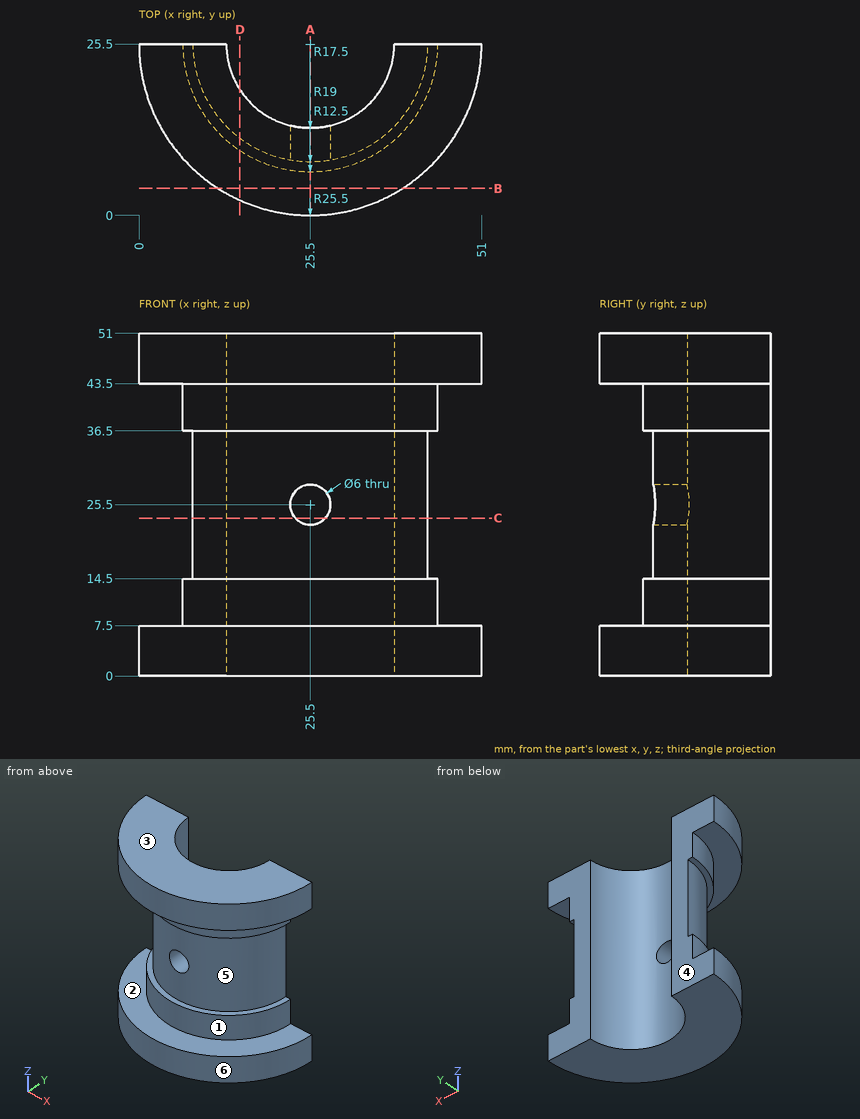
Here's the drawing with two shaded views (mm, measured from the low corner). I have some questions. A direction names the side the tool comes from. Coordinates: 2 decimals unless noted, no trailing zeros. Write each loop counter-clockwise with the first axis right and the second up, starting at its lowest first coordinate (ties: lowest second). Pieces come first, ordered by that corner, then holes.
Item 1: On a 3-axis mill with a long thin cutter (end or side, diameter ignored), from which of +Z, -Z, +X, -X, +Y, -Y can I reach the whole of each face in a straight line? I mean the marked faces 5 and 6. Say none if no direction works.
Item 2: If I drill on line 1 (Z direction, x = 7, y = 8.5); line 2 (Z direction, x = 25.5, y = 11.85); line 3 (Y direction, x = 2.5, z = 5), over which ranges is the centre line in solid material (lowest first)?
Item 3: If we mould it in two halves opening along Z, with no side actions, what happens to the marked faces 1, 2, 3 and 4? For each: +Z half, -Z half, draft (parallel to the pull), parting line (faces both ways), or undercut.
Item 4: I want a section at B-B on y = 4. Write out the boundary of the cut face in (x, z).
Item 5: I want a section at D-D on x = 15. Write out the boundary of the cut face in (y, z), and give its area (3 significant figures).
Item 6: Will these pins go through, and if not, where does the flat tip stop? pin 1 (2 mm diameter, centred on x = 19, z = 31.5, fed in from -Y); pin 2 (8 mm diameter, centred on y = 21, z = 41, fed in from +X); pin 3 (6 mm diameter, centred on x = 45.5, z = 36, fed in from -Y).
Item 7: I want a section at C-C on z = 23.5. Write out the boundary of the cut face in (x, y), and give its area (3 significant figures).
Item 8: I want a section at A-A on x = 25.5. Write out the boundary of the cut face in (y, z).
Findings below:
1. face 5: -Y
1. face 6: +Z, -Z, -Y
2. line 1: z = 0 to 7.5, 43.5 to 51
2. line 2: z = 0 to 22.5, 28.5 to 51
2. line 3: y = 14.49 to 25.5
3. face 1: undercut
3. face 2: undercut
3. face 3: +Z half
3. face 4: draft
4. outline: (11.79, 0) - (39.21, 0) - (39.21, 7.5) - (11.79, 7.5) - close; (11.79, 43.5) - (39.21, 43.5) - (39.21, 51) - (11.79, 51) - close
5. outline: (2.26, 0) - (18.72, 0) - (18.72, 51) - (2.26, 51) - (2.26, 43.5) - (9.66, 43.5) - (9.66, 36.5) - (11.5, 36.5) - (11.5, 14.5) - (9.66, 14.5) - (9.66, 7.5) - (2.26, 7.5) - close
5. area: 532 mm2
6. pin 1: stops at y = 8.89
6. pin 2: stops at x = 50.96
6. pin 3: stops at y = 17.1
7. outline: (8, 25.5) arc R17.5 ccw to (23.26, 8.14) - (23.26, 13.2) arc R12.5 cw to (13, 25.5) - close; (27.74, 8.14) arc R17.5 ccw to (43, 25.5) - (38, 25.5) arc R12.5 cw to (27.74, 13.2) - close
7. area: 213 mm2
8. outline: (0, 0) - (13, 0) - (13, 22.5) - (8, 22.5) - (8, 14.5) - (6.5, 14.5) - (6.5, 7.5) - (0, 7.5) - close; (0, 43.5) - (6.5, 43.5) - (6.5, 36.5) - (8, 36.5) - (8, 28.5) - (13, 28.5) - (13, 51) - (0, 51) - close
